Source: CAD feature listing. Evaluate the final solid. Frame: model axes, mm. Face numbers are marked on the shaded views. A direction names the side the tool comes from. Give positions to 0.01 mm unless a question says otherwise; leave off trailing zeros. Write each loop counter-clockwise with the first axis right and the second up, starting at its lowest first coordinate (ties: lowest second). Pieces come first, ordered by that corner, then holes. Notation, with made-up numbers: M -8.5,58.5 L 8.5,58.5 A16 ccw 8.5,65.5 Z; hole C 19.25,36 d3. An arc over 180 degrees is marked long. Return JSON: item names as keys, results as strings.
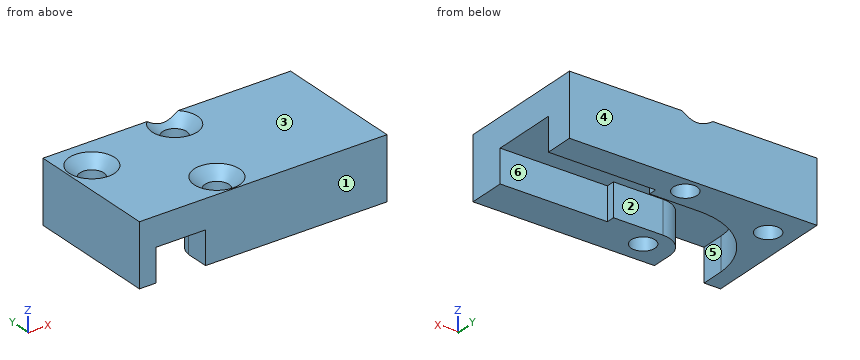
```python
from build123d import *

# Parameters (mm, degrees)
BOSS_EXTRUDE1_DEPTH                                  = 4
BOSS_EXTRUDE1_2_DEPTH                                = 4
SKETCH2_W                                            = 30
SKETCH2_H                                            = 16
BOSS_EXTRUDE2_DEPTH                                  = 3.5
CSK_FOR_M2_5_COUNTERSUNK_FLAT_HEAD_SCREW_D           = 2.9
CSK_FOR_M2_5_COUNTERSUNK_FLAT_HEAD_SCREW_CSINK_D     = 5.5
CSK_FOR_M2_5_COUNTERSUNK_FLAT_HEAD_SCREW_CSINK_ANGLE = 90


with BuildPart() as part:
    # Sketch1 → Boss-Extrude1 (new body)
    with BuildSketch(Plane.XY.offset(0.579115056)):
        with BuildLine():
            Line((110.394950361, -18.30613426), (116.394950361, -18.30613426))
            Line((116.394950361, -18.30613426), (116.394950361, -19.30613426))
            Line((116.394950361, -19.30613426), (129.394950361, -19.30613426))
            Line((129.394950361, -19.30613426), (129.394950361, -23.80613426))
            Line((129.394950361, -23.80613426), (107.399951751, -23.80613426))
            Line((107.399951751, -23.80613426), (107.399951751, -21.00613426))
            ThreePointArc((107.399951751, -21.00613426), (108.376172059, -19.077900974), (110.394950361, -18.30613426))
        make_face()
    extrude(amount=BOSS_EXTRUDE1_DEPTH)



with BuildPart() as body_2:
    # Sketch1 → Boss-Extrude1 2 (new body)
    with BuildSketch(Plane.XY.offset(0.579115056)):
        with BuildLine():
            Line((101.399951751, -21.00613426), (101.399951751, -23.80613426))
            Line((101.399951751, -23.80613426), (99.394950361, -23.80613426))
            Line((99.394950361, -23.80613426), (99.394950361, -7.80613426))
            Line((99.394950361, -7.80613426), (129.394950361, -7.80613426))
            Line((129.394950361, -7.80613426), (129.394950361, -11.30613426))
            Line((129.394950361, -11.30613426), (116.394950361, -11.30613426))
            Line((116.394950361, -11.30613426), (116.394950361, -12.30613426))
            Line((116.394950361, -12.30613426), (110.394950361, -12.30613426))
            ThreePointArc((110.394950361, -12.30613426), (104.137954277, -14.836976664), (101.399951751, -21.00613426))
        make_face()
    extrude(amount=BOSS_EXTRUDE1_2_DEPTH)


with BuildPart() as part_1:
    add(part.part)

    add(body_2.part)  # Boss-Extrude2 merges body 2
    # Sketch2 → Boss-Extrude2 (add)
    with BuildSketch(Plane.XY.offset(4.579115056)):
        with Locations((114.394950361, -15.80613426)):
            Rectangle(SKETCH2_W, SKETCH2_H)
    extrude(amount=BOSS_EXTRUDE2_DEPTH)

    # CSK for M2.5 Countersunk Flat Head Screw1 (through all)
    with Locations(Plane.XY.offset(8.079115056)):
        with Locations((102.394950361, -11.80613426), (113.894950361, -9.80613426), (110.899951751, -20.90613426)):
            CounterSinkHole(CSK_FOR_M2_5_COUNTERSUNK_FLAT_HEAD_SCREW_D / 2, CSK_FOR_M2_5_COUNTERSUNK_FLAT_HEAD_SCREW_CSINK_D / 2, counter_sink_angle=CSK_FOR_M2_5_COUNTERSUNK_FLAT_HEAD_SCREW_CSINK_ANGLE)


solid = part_1.part
```
1) Set-up query: the marked faces 4, 5 and 6. Return all of +Z, -Z, +X, -X, +Y, -Y with unobstructed straight access to the full face (end or side cutting, diameter ignored); none if empty.
Numbers:
{"face 4": "+Z, -Z, +X, -X, +Y", "face 5": "-Z, -Y", "face 6": "-Z, +X"}
2) Contact query for flat-ended pins moving along their axis: pin 1 Ø4.5 at (x, y) = (113.89, -9.81) entering from +Z; pin 2 Ø4 at (x, y) = (115.5, -15) entering from -Z; pin 3 Ø0.5 at (y, z) = (-19, 2) entering from +X. Output: stop coordinate, or through.
Numbers:
{"pin 1": "stops at z = 7.59", "pin 2": "stops at z = 4.58", "pin 3": "stops at x = 116.39"}
3) Line query: line 1 (Y direction, x = 115.5, z = 3); line 2 (Y direction, x = 127, z = 4); line 3 (X direction, y = -20.25, z = 2.25). Output: solid intervals per line, ascending. Write a range as [from, to].
Numbers:
{"line 1": "y = [-23.81, -18.31], [-12.31, -7.81]", "line 2": "y = [-23.81, -19.31], [-11.31, -7.81]", "line 3": "x = [99.39, 101.46], [107.58, 109.61], [112.19, 129.39]"}
4) Cut plane B-B, the plane x = 117. Return the cut outline in (y, z).
Numbers:
{"outline": "M -23.81,0.58 L -19.31,0.58 L -19.31,4.58 L -11.31,4.58 L -11.31,0.58 L -7.81,0.58 L -7.81,8.08 L -23.81,8.08 Z"}
5) Cut plane C-C, the plane z = 7.75. Return the cut outline in (x, y).
Numbers:
{"outline": "M 99.39,-23.81 L 129.39,-23.81 L 129.39,-7.81 L 115.26,-7.81 A2.42 cw long 112.53,-7.81 L 99.39,-7.81 Z; hole C 102.39,-11.81 d4.84; hole C 110.9,-20.91 d4.84"}
6) Cut plane A-A, the plane z = 4.25. Return the cut outline in (x, y), then the cut area to 3 significant figures.
Numbers:
{"outline": "M 99.39,-23.81 L 101.4,-23.81 L 101.4,-21.01 A9 cw 110.39,-12.31 L 116.39,-12.31 L 116.39,-11.31 L 129.39,-11.31 L 129.39,-7.81 L 99.39,-7.81 Z; M 107.4,-23.81 L 129.39,-23.81 L 129.39,-19.31 L 116.39,-19.31 L 116.39,-18.31 L 110.39,-18.31 A3 ccw 107.4,-21.01 Z; hole C 102.39,-11.81 d2.9; hole C 110.9,-20.91 d2.9; hole C 113.89,-9.81 d2.9", "area": "249 mm²"}
7) Draft query along Y for the marked faces 1, 2 and 3. Return one class per face: released by +Y, released by -Y, zero draft, split by the parting line, or undercut.
Numbers:
{"face 1": "released by -Y", "face 2": "undercut", "face 3": "zero draft"}
8) Cut plane D-D, the plane y = -17. Return the cut outline in (x, z).
Numbers:
{"outline": "M 99.39,0.58 L 102.49,0.58 L 102.49,4.58 L 129.39,4.58 L 129.39,8.08 L 99.39,8.08 Z"}
